Part print with two shaded views. Sizes in mm from the minimum x, y, z corner. A direction names the side the tool comes from. Give positions to 0.01 mm unless a question says otherwise; leave off trailing zeros. Loops run counter-clockwise (first coordinate to the right, second up) from the corner with the lowest first, then second, coordinate; pieces in that order, holes last. Notation, with made-up numbers: (79.25, -37) -> (86.25, -37) arc R14 ccw to (86.25, -19) -> close; hole circle Ø8 at (-28.75, 35.5). An arc over 180 degrees is marked (long way). One line per question, with ' | ' between items. Start each with the question number.
(1) Slice it at C-C, the plane y = 31. Write the cut outline in (x, z).
(2) Flat gauge pins, fed straight in: pin 1 Ø1.6 at (x, z) = (30.5, 6.5) entering from +Y; pin 2 Ø4 at (y, z) = (12.5, 2.5) entering from -X; pin 3 Ø4 at (x, z) = (14, 6) entering from -Y. Where does each tip first touch, or does it go through?
(3) 3-axis set-ups, long thin cutter, end or side, ignore diameter. For the marked faces 1 and 2: which of +Z, -Z, +X, -X, +Y, -Y reach the whole face in a straight line?
(4) Slice it at A-A, the plane x = 25. Write the cut outline in (y, z), then the cut area to 4 significant figures.
(5) Slice it at D-D, the plane x = 46.5. Write the cut outline in (y, z), then the cut area to 3 significant figures.
(6) Slice it at B-B, the plane z = 6.5. Write the cut outline in (x, y), then the cut area to 4 significant figures.
(7) Drill centre lines: L1, parallel to Z at x = 33, y = 60; L2, parallel to Y at x = 42, z = 4.25; L3, parallel to Y at x = 28.5, z = 6.5. Where is each one in solid material? Low to high. Write a range as from..to.
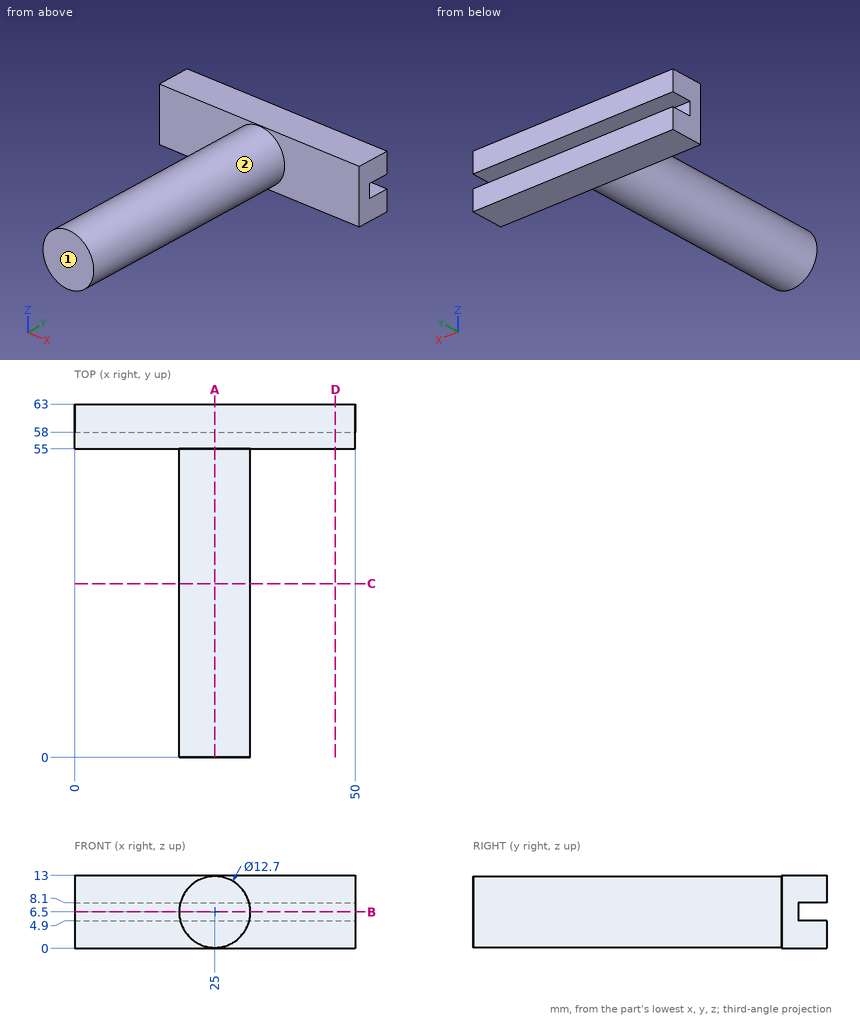
Final values:
1) outline: circle Ø12.7 at (25, 6.5)
2) pin 1: y = 58 | pin 2: x = 18.97 | pin 3: y = 55
3) face 1: +Z, -Z, +X, -X, -Y | face 2: -Y
4) outline: (0, 0.15) -> (55, 0.15) -> (55, 0) -> (63, 0) -> (63, 4.9) -> (58, 4.9) -> (58, 8.1) -> (63, 8.1) -> (63, 13) -> (55, 13) -> (55, 12.85) -> (0, 12.85) -> close | area: 786.5 mm2
5) outline: (55, 0) -> (63, 0) -> (63, 4.9) -> (58, 4.9) -> (58, 8.1) -> (63, 8.1) -> (63, 13) -> (55, 13) -> close | area: 88.0 mm2
6) outline: (0, 55) -> (18.65, 55) -> (18.65, 0) -> (31.35, 0) -> (31.35, 55) -> (50, 55) -> (50, 58) -> (0, 58) -> close | area: 848.5 mm2
7) L1: 0..4.9, 8.1..13 | L2: 55..63 | L3: 0..58
